```python
from build123d import *

# Parameters (mm, degrees)
SKETCH2_R           = 2.667
BOSS_EXTRUDE1_DEPTH = 6.35
BOSS_EXTRUDE2_DEPTH = 38.1
CUT_EXTRUDE1_DEPTH  = 50.8
CUT_EXTRUDE2_DEPTH  = 38.1
BOSS_EXTRUDE3_DEPTH = 9.525
BOSS_EXTRUDE4_DEPTH = 6.35
BOSS_EXTRUDE5_DEPTH = 22.225
CUT_EXTRUDE4_DEPTH  = 19.05
CUT_EXTRUDE7_DEPTH  = 19.05
CUT_EXTRUDE8_DEPTH  = 6.35
CUT_EXTRUDE9_DEPTH  = 6.35


with BuildPart() as part:
    # Sketch2 → Boss-Extrude1 (new body)
    with BuildSketch(Plane(origin=(0, 0, 0), x_dir=(1, 0, 0), z_dir=(0, 1, 0))):
        with BuildLine():
            Line((-109.5375, -9.525), (-109.5375, -61.948583794))
            ThreePointArc((-109.5375, -61.948583794), (-108.60756403, -64.193647824), (-106.3625, -65.123583794))
            Line((-106.3625, -65.123583794), (-100.0125, -65.123583794))
            ThreePointArc((-100.0125, -65.123583794), (-97.76743597, -64.193647824), (-96.8375, -61.948583794))
            Line((-96.8375, -61.948583794), (-96.8375, -34.925))
            ThreePointArc((-96.8375, -34.925), (-95.90756403, -32.67993597), (-93.6625, -31.75))
            Line((-93.6625, -31.75), (-28.575, -31.75))
            ThreePointArc((-28.575, -31.75), (-26.32993597, -32.67993597), (-25.4, -34.925))
            Line((-25.4, -34.925), (-25.4, -61.948583794))
            ThreePointArc((-25.4, -61.948583794), (-24.47006403, -64.193647824), (-22.225, -65.123583794))
            Line((-22.225, -65.123583794), (-9.525, -65.123583794))
            ThreePointArc((-9.525, -65.123583794), (-7.27993597, -64.193647824), (-6.35, -61.948583794))
            Line((-6.35, -61.948583794), (-6.35, -12.7))
            ThreePointArc((-6.35, -12.7), (-8.209871939, -8.209871939), (-12.7, -6.35))
            Line((-12.7, -6.35), (-106.3625, -6.35))
            ThreePointArc((-106.3625, -6.35), (-108.60756403, -7.27993597), (-109.5375, -9.525))
        make_face()
        with Locations((-95.25, -16.637060646)):
            Circle(SKETCH2_R, mode=Mode.SUBTRACT)
        with Locations((-31.75, -16.637060646)):
            Circle(SKETCH2_R, mode=Mode.SUBTRACT)
    extrude(amount=-BOSS_EXTRUDE1_DEPTH)

    # Sketch3 → Boss-Extrude2 (add)
    with BuildSketch(Plane.XZ.offset(6.35)):
        with BuildLine():
            Line((-6.35, 61.948583794), (-6.35, 12.7))
            ThreePointArc((-6.35, 12.7), (-8.209871939, 8.209871939), (-12.7, 6.35))
            Line((-12.7, 6.35), (-96.8375, 6.35))
            Line((-96.8375, 6.35), (-96.8375, 12.7))
            Line((-96.8375, 12.7), (-88.9, 12.7))
            Line((-88.9, 12.7), (-88.9, 31.75))
            Line((-88.9, 31.75), (-82.55, 31.75))
            Line((-82.55, 31.75), (-82.55, 12.7))
            Line((-82.55, 12.7), (-66.675, 12.7))
            Line((-66.675, 12.7), (-66.675, 31.75))
            Line((-66.675, 31.75), (-60.325, 31.75))
            Line((-60.325, 31.75), (-60.325, 12.7))
            Line((-60.325, 12.7), (-44.45, 12.7))
            Line((-44.45, 12.7), (-44.45, 31.75))
            Line((-44.45, 31.75), (-38.1, 31.75))
            Line((-38.1, 31.75), (-38.1, 12.7))
            Line((-38.1, 12.7), (-15.875, 12.7))
            ThreePointArc((-15.875, 12.7), (-13.62993597, 13.62993597), (-12.7, 15.875))
            Line((-12.7, 15.875), (-12.7, 27.023583794))
            Line((-12.7, 27.023583794), (-25.4, 27.023583794))
            Line((-25.4, 27.023583794), (-25.4, 33.373583794))
            Line((-25.4, 33.373583794), (-12.7, 33.373583794))
            Line((-12.7, 33.373583794), (-12.7, 42.898583794))
            Line((-12.7, 42.898583794), (-25.4, 42.898583794))
            Line((-25.4, 42.898583794), (-25.4, 49.248583794))
            Line((-25.4, 49.248583794), (-12.7, 49.248583794))
            Line((-12.7, 49.248583794), (-12.7, 58.773583794))
            Line((-12.7, 58.773583794), (-25.4, 58.773583794))
            Line((-25.4, 58.773583794), (-25.4, 61.948583794))
            ThreePointArc((-25.4, 61.948583794), (-24.47006403, 64.193647824), (-22.225, 65.123583794))
            Line((-22.225, 65.123583794), (-9.525, 65.123583794))
            ThreePointArc((-9.525, 65.123583794), (-7.27993597, 64.193647824), (-6.35, 61.948583794))
        make_face()
    extrude(amount=BOSS_EXTRUDE2_DEPTH)

    # Sketch4 → Cut-Extrude1 (cut)
    with BuildSketch(Plane.ZY.offset(88.9)):
        Polygon((31.75, -6.35), (12.7, -44.45), (31.75, -44.45), align=None)
    extrude(amount=-CUT_EXTRUDE1_DEPTH, mode=Mode.SUBTRACT)

    # Sketch5 → Cut-Extrude2 (cut)
    with BuildSketch(Plane.XY.offset(65.123583794)):
        Polygon((-25.4, -6.35), (-12.7, -44.45), (-25.4, -44.45), align=None)
    extrude(amount=-CUT_EXTRUDE2_DEPTH, mode=Mode.SUBTRACT)

    # Sketch6 → Boss-Extrude3 (add)
    with BuildSketch(Plane.XZ.offset(6.35)):
        with BuildLine():
            Line((-96.8375, 6.35), (-106.3625, 6.35))
            ThreePointArc((-106.3625, 6.35), (-108.60756403, 7.27993597), (-109.5375, 9.525))
            Line((-109.5375, 9.525), (-109.5375, 61.948583794))
            ThreePointArc((-109.5375, 61.948583794), (-108.60756403, 64.193647824), (-106.3625, 65.123583794))
            Line((-106.3625, 65.123583794), (-100.0125, 65.123583794))
            ThreePointArc((-100.0125, 65.123583794), (-97.76743597, 64.193647824), (-96.8375, 61.948583794))
            Line((-96.8375, 61.948583794), (-96.8375, 6.35))
        make_face()
    extrude(amount=BOSS_EXTRUDE3_DEPTH)

    # Sketch7 → Boss-Extrude4 (add)
    with BuildSketch(Plane.XZ.offset(15.875)):
        with BuildLine():
            Line((-100.0125, 65.123583794), (-138.1125, 65.123583794))
            ThreePointArc((-138.1125, 65.123583794), (-140.35756403, 64.193647824), (-141.2875, 61.948583794))
            Line((-141.2875, 61.948583794), (-141.2875, 19.05))
            ThreePointArc((-141.2875, 19.05), (-137.567756121, 10.069743879), (-128.5875, 6.35))
            Line((-128.5875, 6.35), (-96.8375, 6.35))
            Line((-96.8375, 6.35), (-96.8375, 61.948583794))
            ThreePointArc((-96.8375, 61.948583794), (-97.76743597, 64.193647824), (-100.0125, 65.123583794))
        make_face()
    extrude(amount=BOSS_EXTRUDE4_DEPTH)

    # Sketch8 → Boss-Extrude5 (add)
    with BuildSketch(Plane.XZ.offset(22.225)):
        with BuildLine():
            Line((-128.5875, 6.35), (-96.8375, 6.35))
            Line((-96.8375, 6.35), (-96.8375, 12.7))
            Line((-96.8375, 12.7), (-96.8375, 38.1))
            Line((-96.8375, 38.1), (-134.9375, 38.1))
            Line((-134.9375, 38.1), (-134.9375, 46.073583794))
            Line((-134.9375, 46.073583794), (-96.8375, 46.073583794))
            Line((-96.8375, 46.073583794), (-96.8375, 52.423583794))
            Line((-96.8375, 52.423583794), (-134.9375, 52.423583794))
            Line((-134.9375, 52.423583794), (-134.9375, 58.773583794))
            Line((-134.9375, 58.773583794), (-96.8375, 58.773583794))
            Line((-96.8375, 58.773583794), (-96.8375, 61.948583794))
            ThreePointArc((-96.8375, 61.948583794), (-97.76743597, 64.193647824), (-100.0125, 65.123583794))
            Line((-100.0125, 65.123583794), (-138.1125, 65.123583794))
            ThreePointArc((-138.1125, 65.123583794), (-140.35756403, 64.193647824), (-141.2875, 61.948583794))
            Line((-141.2875, 61.948583794), (-141.2875, 19.05))
            ThreePointArc((-141.2875, 19.05), (-137.567756121, 10.069743879), (-128.5875, 6.35))
        make_face()
        with BuildLine():
            Line((-128.5875, 12.7), (-103.1875, 12.7))
            Line((-103.1875, 12.7), (-103.1875, 31.75))
            Line((-103.1875, 31.75), (-134.9375, 31.75))
            Line((-134.9375, 31.75), (-134.9375, 19.05))
            ThreePointArc((-134.9375, 19.05), (-133.07762806, 14.559871939), (-128.5875, 12.7))
        make_face(mode=Mode.SUBTRACT)
    extrude(amount=BOSS_EXTRUDE5_DEPTH)

    # Sketch11 → Cut-Extrude4 (cut)
    with BuildSketch(Plane.XY.offset(65.123583794)):
        Polygon((-134.9375, -44.45), (-96.8375, -22.225), (-96.8375, -44.45), align=None)
    extrude(amount=-CUT_EXTRUDE4_DEPTH, mode=Mode.SUBTRACT)

    # Sketch23 → Cut-Extrude7 (cut)
    with BuildSketch(Plane(origin=(-0.256512778, 0.439736191, -0.384769167), x_dir=(0.915651215, 0.302516036, -0.264701531), z_dir=(-0.401973696, 0.689097765, -0.602960544))):
        Polygon((-105.477921765, 19.712805797), (-105.477921765, -14.037907158), (-147.087651949, 0.597357751), align=None)
    extrude(amount=-CUT_EXTRUDE7_DEPTH, mode=Mode.SUBTRACT)

    # Sketch24 → Cut-Extrude8 (cut)
    with BuildSketch(Plane.ZY.offset(103.1875)):
        Polygon((31.75, -31.485416667), (12.7, -44.45), (16.933333333, -44.45), align=None)
    extrude(amount=-CUT_EXTRUDE8_DEPTH, mode=Mode.SUBTRACT)

    # Sketch25 → Cut-Extrude9 (cut)
    with BuildSketch(Plane(origin=(0, 0, 31.75), x_dir=(-1, 0, 0), z_dir=(0, 0, -1))):
        Polygon((103.1875, -31.485416667), (134.9375, -44.45), (125.4125, -44.45), align=None)
    extrude(amount=-CUT_EXTRUDE9_DEPTH, mode=Mode.SUBTRACT)


solid = part.part
```
Read the model definition and answer for the solid it produces. Units are mm, in the model's axes. A direction names the side the tool comes from. Coordinates: 2 decimals unless noted, no trailing zeros. Write each loop counter-clockwise with the first axis right and the second up, starting at its lowest first coordinate (ties: lowest second). Pieces come first, ordered by that corner, then holes. Notation, with made-up numbers: (35, 37.25) - (42, 37.25) arc R23 ccw to (42, 56.25) - close; hole circle Ø2 at (30.5, 89). An arc over 180 degrees is marked (long way). Answer as a JSON object with one key per item and string values. Group by question number.
1. A cutting plane is placed at A-A (x = -31.75). Determine the outline of the cut face in (y, z).
2. A cutting plane is placed at D-D (x = -95.25). Determine the outline of the cut face in (y, z), plus the area to 3 significant figures.
3. Each of these flat-tipped pins is pushed along its axis until it touches: P1, Ø1, axis at x = -29.5, y = -24.5, coming from the +Z side; P2, Ø12.5, axis at x = -52.5, z = 19.5, coming from the -Y side; P3, Ø3, axis at x = -115, z = 55.5, coming from the -Y side (3 decimals). Where does it stop, or does it pass through?
4. The mould has two halves that part along X. Classify faces 5 (the flat face through (-18, -21, 58.774)), 6 (the cylindrical face through (-140.33, -29.96, 64.22)): +X half, -X half, draft (parallel to the pull), parting line (faces both ways), or undercut.
5. Consider L1, parallel to Z at x = -124.5, y = -28; L2, parallel to X at y = -7.5, z = 56.5; L3, parallel to X at y = -24.5, z = 41.5. Determine where each line is inside the solid, lowest interval first. Write a range as [from, to].
6. Which of the six approach directions +Z, -Z, +X, -X, +Y, -Y give full straight-line access (tool end or side, diameter ignored) to faces 1 (the cylindrical face through (-108.6, -7.8, 64.2)), 2 (the flat face through (-88.9, -21, 20)), 3 (the cylindrical face through (-26.35, -3.13, 32.66)), 4 (the flat face through (-116, -22.225, 56))?
Worked out:
{
 "1": {"outline": "(-44.45, 6.35) - (0, 6.35) - (0, 13.97) - (-6.35, 13.97) - (-6.35, 12.7) - (-44.45, 12.7) - close; (-6.35, 19.3) - (0, 19.3) - (0, 31.75) - (-6.35, 31.75) - close"},
 "2": {"outline": "(-44.45, 6.35) - (0, 6.35) - (0, 13.97) - (-6.35, 13.97) - (-6.35, 12.7) - (-44.45, 12.7) - close; (-6.35, 19.3) - (0, 19.3) - (0, 32.18) - (-6.35, 32.18) - close", "area": "372 mm²"},
 "3": {"P1": "stops at z = 12.7", "P2": "stops at y = -6.35", "P3": "stops at y = -22.225"},
 "4": {"face 5": "undercut", "face 6": "-X half"},
 "5": {"L1": "z = [6.35, 12.7], [31.75, 38.1], [46.07, 52.42], [58.77, 65.12]", "L2": "x = [-109.54, -96.84], [-12.7, -6.35]", "L3": "x = [-141.29, -134.94], [-12.7, -6.35]"},
 "6": {"face 1": "+Z, -X, +Y", "face 2": "+Z, -Y", "face 3": "+Z, +Y, -Y", "face 4": "-Y"}
}
